Design review of the part built by this model. Coordinates are the model's own, in mm. A direction names the side the tool comes from. Coordinates: 2 decimals unless noted, no trailing zeros. Loops run counter-clockwise (first coordinate to the right, second up) from the corner with the lowest first, then second, coordinate; pieces in that order, holes last.
from build123d import *

# Parameters (mm, degrees)
SKETCH_R        = 1.75
PAD_DEPTH       = 4
PAD001_DEPTH    = 25
SKETCH002_W     = 16
SKETCH002_H     = 10
POCKET_DEPTH    = 2
SKETCH003_W     = 16
SKETCH003_H     = 16
POCKET001_DEPTH = 2
SKETCH004_W     = 12
SKETCH004_H     = 8
PAD002_DEPTH    = 8
SKETCH005_W     = 12
SKETCH005_H     = 8
PAD003_DEPTH    = 8
SKETCH006_W     = 5
SKETCH006_H     = 6
POCKET002_DEPTH = 8
SKETCH007_R     = 5
POCKET003_DEPTH = 44.001
SKETCH008_R     = 4
POCKET004_DEPTH = 2


with BuildPart() as part:
    # Sketch → Pad (new body)
    with BuildSketch(Plane.XY):
        Polygon((-21, 21), (21, 21), (21, -21), (18, -21), (18, -69), (-18, -69), (-18, -21), (-21, -21), align=None)
        with Locations((-15, 15)):
            Circle(SKETCH_R, mode=Mode.SUBTRACT)
        with Locations((15, 15)):
            Circle(SKETCH_R, mode=Mode.SUBTRACT)
        with Locations((-15, -15)):
            Circle(SKETCH_R, mode=Mode.SUBTRACT)
        with Locations((15, -15)):
            Circle(SKETCH_R, mode=Mode.SUBTRACT)
    extrude(amount=PAD_DEPTH)

    # Sketch001 (on Face14 of Pad) → Pad001 (join)
    with BuildSketch(Plane.XY.offset(4)):
        Polygon((-21, 21), (21, 21), (21, -21), (18, -21), (18, -69), (-18, -69), (-18, -21), (-21, -21), align=None)
        Polygon((-19, 19), (-19, -19), (-16, -19), (-16, -67), (16, -67), (16, -19), (19, -19), (19, 19), align=None, mode=Mode.SUBTRACT)
    extrude(amount=PAD001_DEPTH)

    # Sketch002 (on Face7 of Pad001) → Pocket (cut)
    with BuildSketch(Plane.XZ.offset(69)):
        with Locations((0, 9)):
            Rectangle(SKETCH002_W, SKETCH002_H)
    extrude(amount=-POCKET_DEPTH, mode=Mode.SUBTRACT)

    # Sketch003 (on Face26 of Pocket) → Pocket001 (cut)
    with BuildSketch(Plane.YZ.offset(21)):
        with Locations((7, 14)):
            Rectangle(SKETCH003_W, SKETCH003_H)
    extrude(amount=-POCKET001_DEPTH, mode=Mode.SUBTRACT)

    # Sketch004 (on Face19 of Pocket001) → Pad002 (join)
    with BuildSketch(Plane.YZ.offset(18)):
        with Locations((-31, 12)):
            Rectangle(SKETCH004_W, SKETCH004_H)
    extrude(amount=PAD002_DEPTH)

    # Sketch005 (on Face5 of Pad002) → Pad003 (join)
    with BuildSketch(Plane(origin=(-18, 0, 0), x_dir=(0, -1, 0), z_dir=(-1, 0, 0))):
        with Locations((31, 12)):
            Rectangle(SKETCH005_W, SKETCH005_H)
    extrude(amount=PAD003_DEPTH)

    # Sketch006 (on Face22 of Pad003) → Pocket002 (cut)
    with BuildSketch(Plane.XY.offset(16)):
        with Locations((-20.5, -31)):
            Rectangle(SKETCH006_W, SKETCH006_H)
        with Locations((20.5, -31)):
            Rectangle(SKETCH006_W, SKETCH006_H)
    extrude(amount=-POCKET002_DEPTH, mode=Mode.SUBTRACT)

    # Sketch007 (on Face24 of Pocket002) → Pocket003 (cut, through all)
    with BuildSketch(Plane.YZ.offset(18)):
        with Locations((-47, 16)):
            Circle(SKETCH007_R)
    extrude(amount=-POCKET003_DEPTH, mode=Mode.SUBTRACT)

    # Sketch008 (on Face4 of Pocket003) → Pocket004 (cut)
    with BuildSketch(Plane(origin=(0, 0, 0), x_dir=(1, 0, 0), z_dir=(0, 0, -1))):
        with Locations((-15, -15)):
            Circle(SKETCH008_R)
        with Locations((-15, 15)):
            Circle(SKETCH008_R)
        with Locations((15, 15)):
            Circle(SKETCH008_R)
        with Locations((15, -15)):
            Circle(SKETCH008_R)
    extrude(amount=-POCKET004_DEPTH, mode=Mode.SUBTRACT)


solid = part.part
Q1. For line 1 (Y direction, x = -15, z = 3.55); line 2 (X direction, y = -15, z = 1.3); line 3 (Y direction, x = -15, z = 0.95), list the stretches that pass through material, from the lowest coordinate up.
Q2. Take a section at B-B, the plane z = 24.75. Write out the cut boundary in (x, y).
Q3. Machinability: for faces 1 (the flat face through (-22, -25, 12)), 2 (the flat face through (0, -67, 19)), 3 (the flat face through (8, -68, 9)), 4 (the flat face through (-14, 17, 2)), 5 (the flat face through (-24, -31, 8)), which of the approach directions +Z, -Z, +X, -X, +Y, -Y give a long, thin tool a straight path to every point of the face, cutting with its end or side? Answer none if there is none.
Q4. Take a section at A-A, the plane y = -47. Write out the cut boundary in (x, z), then the cut area to 3 significant figures.
Q5. Clearance check with flat-ended pins moving along their axes: pin 1 Ø4 at (y, z) = (-46.5, 18) entering from +X; pin 2 Ø8 at (x, y) = (-5, -50.5) entering from +Z; pin 3 Ø4 at (x, y) = (16, -15.5) entering from -Z; pin 4 Ø2.5 at (x, z) = (-19.5, 13.5) entering from -Y. State where each tip first meets the part, or that it passes through.
Q6. The part is to be moulded in two halves that separate along X. For faces 6 (the flat face through (26, -31, 12)), 7 (the flat face through (0, 19, 16)), 8 (the flat face through (20, 7, 6)), say which applies: pulls with the +X half, pulls with the -X half, needs draft (parallel to the pull), parting line crosses it, or undercut.
Q7. Take a section at D-D, the plane z = 15. Give the number of separate pieces and of enclosed holes in the cut face, then the cut area to 3 significant figures.
Q8. Take a section at C-C, the plane x = 15. Write out the cut boundary in (y, z).
Entries:
1. line 1: y = -69 to -16.75, -13.25 to 13.25, 16.75 to 21
1. line 2: x = -21 to -19, -11 to 11, 19 to 21
1. line 3: y = -69 to -19, -11 to 11, 19 to 21
2. outline: (-21, -21) - (-18, -21) - (-18, -69) - (18, -69) - (18, -21) - (21, -21) - (21, 21) - (-21, 21) - close; hole (-19, -19) - (-16, -19) - (-16, -67) - (16, -67) - (16, -19) - (19, -19) - (19, 19) - (-19, 19) - close
3. face 1: +Z, -Z, -X
3. face 2: +Z
3. face 3: -Y
3. face 4: -Z
3. face 5: -Z, -X, -Y
4. outline: (-18, 0) - (18, 0) - (18, 11) - (16, 11) - (16, 4) - (-16, 4) - (-16, 11) - (-18, 11) - close; (-18, 21) - (-16, 21) - (-16, 29) - (-18, 29) - close; (16, 21) - (18, 21) - (18, 29) - (16, 29) - close
4. area: 204 mm2
5. pin 1: passes through
5. pin 2: stops at z = 4
5. pin 3: stops at z = 2
5. pin 4: stops at y = -37
6. face 6: pulls with the +X half
6. face 7: undercut
6. face 8: needs draft
7. separate pieces: 3
7. enclosed holes: 2
7. area: 573 mm2
8. outline: (-69, 0) - (-19, 0) - (-19, 2) - (-16.75, 2) - (-16.75, 4) - (-67, 4) - (-67, 29) - (-69, 29) - close; (-13.25, 2) - (-11, 2) - (-11, 0) - (11, 0) - (11, 2) - (13.25, 2) - (13.25, 4) - (-13.25, 4) - close; (16.75, 2) - (19, 2) - (19, 0) - (21, 0) - (21, 29) - (19, 29) - (19, 4) - (16.75, 4) - close
